Part print with two shaded views. Sizes in mm from the minimum x, y, z corner. Round coordinates to 2 decimals unless told otherwise and drop trailing zeros. Loops run counter-clockwise (first coordinate to the right, second up) from the corner with the lowest first, then second, coordinate; pieces in that order, holes last. Notation, with made-up numbers: (14, 81.25) -> (42, 81.25) arc R27 ccw to (42, 113.25) -> close; hole circle Ø5 at (-25.5, -14). An arc over 180 degrees is marked (long way). Use a Markdown table: item, result. Add a question column.
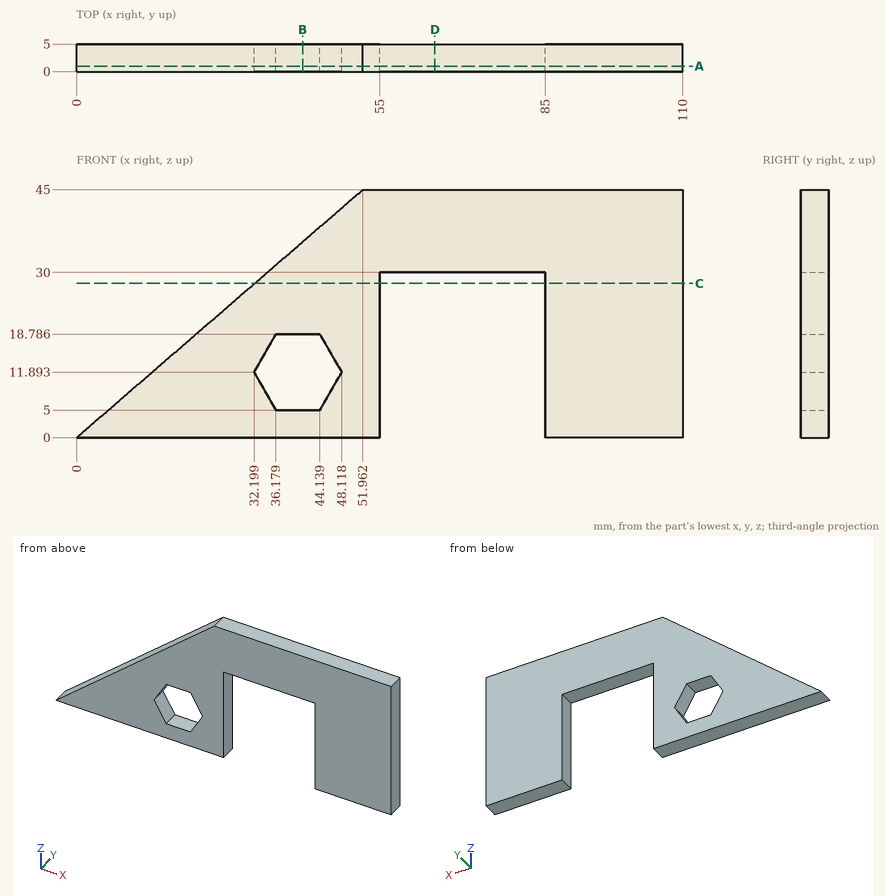
1) Pin check, flat tips, straight feed: pin 1 Ø1 at (y, z) = (3, 14) entering from -X; pin 2 Ø1.5 at (x, z) = (14.5, 6) entering from -Y; pin 3 Ø1.5 at (y, z) = (3.5, 16.5) entering from -X (1 decimal); pin 4 Ø1.5 at (x, y) = (44.5, 1) entering from +Z. Stop position of each tip, or through.
2) Cut at C-C on z = 28. Write the cut outline in (x, y), and give its area (3 significant figures).
3) Cut at A-A on y = 1. Write the cut outline in (x, z), and give its area (3 significant figures).
4) Cut at B-B on x = 41. Write the cut outline in (y, z), and give its area (3 significant figures).
5) Cut at D-D on x = 65. Write the cut outline in (y, z), and give its area (3 significant figures).
6) Wall check: probe 1 along X at (y, z) = (0.45, 13.5) (1 decimal); probe 2 along X at (y, z) = (3.85, 6) (1 decimal); probe 3 along Z at (x, y) = (68.5, 1.05). Give the ranges that are in metal, low to high. Write a range as from..to.
Established:
| question | item | result |
|---|---|---|
| 1 | pin 1 | stops at x = 15.59 |
| 1 | pin 2 | stops at y = 0 |
| 1 | pin 3 | stops at x = 18.2 |
| 1 | pin 4 | stops at z = 39.19 |
| 2 | outline | (32.33, 0) -> (55, 0) -> (55, 5) -> (32.33, 5) -> close; (85, 0) -> (110, 0) -> (110, 5) -> (85, 5) -> close |
| 2 | area | 238 mm^2 |
| 3 | outline | (0, 0) -> (55, 0) -> (55, 30) -> (85, 30) -> (85, 0) -> (110, 0) -> (110, 45) -> (51.96, 45) -> close; hole (32.2, 11.89) -> (36.18, 5) -> (44.14, 5) -> (48.12, 11.89) -> (44.14, 18.79) -> (36.18, 18.79) -> close |
| 3 | area | 2,720 mm^2 |
| 4 | outline | (0, 0) -> (5, 0) -> (5, 5) -> (0, 5) -> close; (0, 18.79) -> (5, 18.79) -> (5, 35.51) -> (0, 35.51) -> close |
| 4 | area | 109 mm^2 |
| 5 | outline | (0, 30) -> (5, 30) -> (5, 45) -> (0, 45) -> close |
| 5 | area | 75.0 mm^2 |
| 6 | probe 1 | x = 15.6..33.1, 47.2..55, 85..110 |
| 6 | probe 2 | x = 6.9..35.6, 44.7..55, 85..110 |
| 6 | probe 3 | z = 30..45 |
